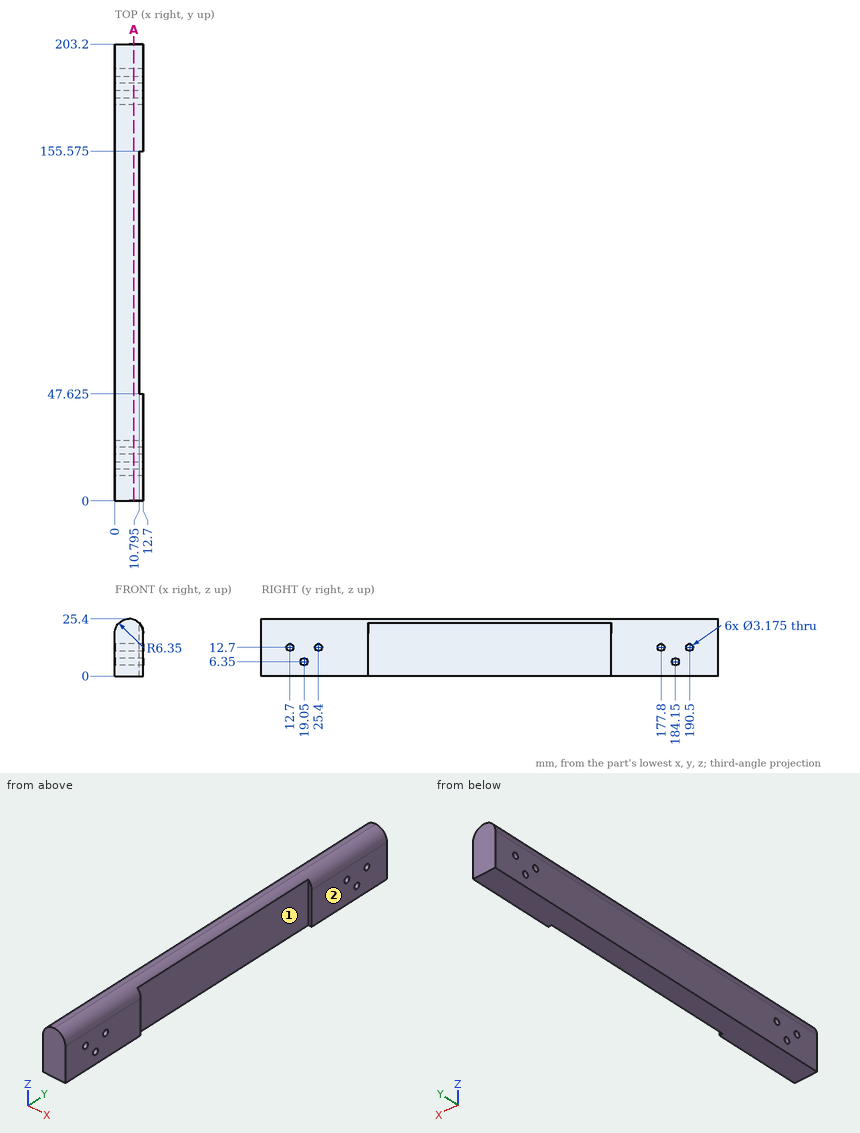
Can you work these out from the drawing? Everything is in mm from the part's minimum corner. A direction names the side the tool comes from. Coordinates: 2 decimals unless noted, no trailing zeros. Answer as CSV lines item,"result". Start each with the question number.
1. I want a section at A-A, the plane x = 8.5. Count the separate pieces of the cut face and the enclosed holes in it, and give its area (3 significant figures).
2. I need wall thicknesses on line 1 (X direction, y = 134, z = 17.5) (3 decimals); line 2 (Z direction, x = 6.25, y = 115); line 3 (Z direction, x = 4, y = 184.15). Which ranges of each line are inside material? Lowest first, please. Write a range as [from, to].
3. On a 3-axis mill with a long thin cutter (end or side, diameter ignored), from which of +Z, -Z, +X, -X, +Y, -Y can I reach the whole of each face in a straight line? I mean the marked faces 1 and 2. Say none if no direction works.
4. For pin 1 (1.9 mm diameter, centred on y = 19.05, z = 6.35, fed in from +X); pin 2 (4 mm diameter, centred on y = 121, z = 7.5, fed in from +X) (3 decimals), each with a flat end and sliding along its axis, tell me the tip position at first contact or that it passes through.
Recorded:
1,separate pieces,"1"
1,enclosed holes,"6"
1,area,"5,040 mm2"
2,line 1,"x = [0, 10.795]"
2,line 2,"z = [0, 25.4]"
2,line 3,"z = [0, 4.76], [7.94, 24.95]"
3,face 1,"+Z, -Z, +X"
3,face 2,"+Z, -Z, +X, +Y, -Y"
4,pin 1,"passes through"
4,pin 2,"stops at x = 10.795"
